Design review of the part built by this model. Coordinates are the model's own, in mm. A direction names the side the tool comes from. Give positions to 0.01 mm unless a question says otherwise; leave off trailing zeros. Order: outer loops, then holes, each group sorted by start corner. A loop starts at its lowest first (then second) coordinate and runs counter-clockwise, first axis right, second up. Notation, with made-up numbers: (16.25, 37.5) -> (42.25, 37.5) arc R7 cw to (42.25, 47.5) -> close; hole circle Ø11 at (42, 53). An arc over 180 degrees is marked (long way). One line per item, written item: value.
from build123d import *

# Parameters (mm, degrees)
SKETCH_1_W               = 45
SKETCH_1_H               = 12
EXTRUDE_1_DEPTH          = 4
SKETCH_2_W               = 12
SKETCH_2_H               = 12
EXTRUDE_2_DEPTH          = 15
SKETCH_3_W               = 2
SKETCH_3_H               = 10
EXTRUDE_3_DEPTH          = 2
SKETCH_4_W               = 21
SKETCH_4_H               = 21
EXTRUDE_4_DEPTH          = 19
SKETCH_5_W               = 13
SKETCH_5_H               = 13
CUT_EXTRUDE_1_DEPTH      = 50.782024868
SKETCH_6_W               = 13
SKETCH_6_H               = 4
CUT_EXTRUDE_2_DEPTH      = 12
CUT_EXTRUDE_3_REACH      = 54.671
SKETCH_7_W               = 5
SKETCH_7_H               = 2
CUT_EXTRUDE_4_REACH      = 54.671
SKETCH_8_R               = 1.5
CHAMFER_1_SIZE           = 2
CUT_EXTRUDE_5_DEPTH      = 50.053542176
CUT_EXTRUDE_5_DEPTH_BACK = 50.053542176
SKETCH_9_R               = 3.5
CUT_EXTRUDE_6_DEPTH      = 51.5791459
CUT_EXTRUDE_6_DEPTH_BACK = 2
SKETCH_10_R              = 2
CUT_EXTRUDE_7_DEPTH      = 50.782024868
CUT_EXTRUDE_7_DEPTH_BACK = 50.782024868
SKETCH_11_R              = 2
CUT_EXTRUDE_8_DEPTH      = 51.5791459
CUT_EXTRUDE_8_DEPTH_BACK = 10
SKETCH_12_R              = 3.5
SKETCH_13_W              = 21
SKETCH_13_H              = 7
CUT_EXTRUDE_9_DEPTH      = 17
SKETCH_14_R              = 3.5
EXTRUDE_5_DEPTH          = 4


with BuildPart() as part:
    # 草图1 → 凸台-拉伸1 (new body)
    with BuildSketch(Plane(origin=(0, 0, 0), x_dir=(1, 0, 0), z_dir=(0, 1, 0))):
        Rectangle(SKETCH_1_W, SKETCH_1_H)
    extrude(amount=EXTRUDE_1_DEPTH)

    # 草图2 → 凸台-拉伸2 (add)
    with BuildSketch(Plane(origin=(0, 4, 0), x_dir=(1, 0, 0), z_dir=(0, 1, 0))):
        with Locations((16.5, 0)):
            Rectangle(SKETCH_2_W, SKETCH_2_H)
    extrude(amount=EXTRUDE_2_DEPTH)

    # 草图3 → 凸台-拉伸3 (add)
    with BuildSketch(Plane(origin=(0, 19, 0), x_dir=(1, 0, 0), z_dir=(0, 1, 0))):
        with Locations((11.5, 0)):
            Rectangle(SKETCH_3_W, SKETCH_3_H)
        with Locations((21.5, 0)):
            Rectangle(SKETCH_3_W, SKETCH_3_H)
    extrude(amount=EXTRUDE_3_DEPTH)

    # 草图4 → 凸台-拉伸4 (add)
    with BuildSketch(Plane.XZ):
        with Locations((33, -4.5)):
            Rectangle(SKETCH_4_W, SKETCH_4_H)
    extrude(amount=-EXTRUDE_4_DEPTH)

    # 草图5 → 切除-拉伸1 (cut, through all)
    with BuildSketch(Plane(origin=(0, 19, 0), x_dir=(1, 0, 0), z_dir=(0, 1, 0))):
        with Locations((33, 4.5)):
            Rectangle(SKETCH_5_W, SKETCH_5_H)
    extrude(amount=-CUT_EXTRUDE_1_DEPTH, mode=Mode.SUBTRACT)

    # 草图6 → 切除-拉伸2 (cut)
    with BuildSketch(Plane(origin=(0, 19, 0), x_dir=(1, 0, 0), z_dir=(0, 1, 0))):
        with Locations((33, -4)):
            Rectangle(SKETCH_6_W, SKETCH_6_H)
    extrude(amount=-CUT_EXTRUDE_2_DEPTH, mode=Mode.SUBTRACT)

    # 草图7 → 切除-拉伸3 (cut, up to next)
    with BuildSketch(Plane.XY.offset(6), mode=Mode.PRIVATE) as cut_extrude_3_sk1:
        with Locations((33, 7)):
            Rectangle(SKETCH_7_W, SKETCH_7_H)
    cut_extrude_3_tool1 = extrude(cut_extrude_3_sk1.sketch, amount=-CUT_EXTRUDE_3_REACH, mode=Mode.PRIVATE) & part.part
    add(cut_extrude_3_tool1.solids().sort_by_distance((33, 7, 6))[0], mode=Mode.SUBTRACT)

    # 草图8 → 切除-拉伸4 (cut, up to next)
    with BuildSketch(Plane.XY.offset(6), mode=Mode.PRIVATE) as cut_extrude_4_sk1:
        with Locations((33, 4)):
            Circle(SKETCH_8_R)
    cut_extrude_4_tool1 = extrude(cut_extrude_4_sk1.sketch, amount=-CUT_EXTRUDE_4_REACH, mode=Mode.PRIVATE) & part.part
    add(cut_extrude_4_tool1.solids().sort_by_distance((33, 4, 6))[0], mode=Mode.SUBTRACT)

    # 倒角1
    chamfer_1_edges = [part.edges().sort_by_distance(p)[0] for p in [
        (-22.5, 2, -6),
        (-22.5, 2, 6),
    ]]
    chamfer(chamfer_1_edges, length=CHAMFER_1_SIZE)

    # 草图9 → 切除-拉伸5 (cut, two sides: drawn at the far end of the back side and taken through both)
    with BuildSketch(Plane(origin=(0, 4, 0), x_dir=(1, 0, 0), z_dir=(0, 1, 0)).offset(-CUT_EXTRUDE_5_DEPTH_BACK)):
        with Locations(Location((-15.5, 0, 0), (0, 0, 270))):
            Circle(SKETCH_9_R)
    extrude(amount=CUT_EXTRUDE_5_DEPTH + CUT_EXTRUDE_5_DEPTH_BACK, mode=Mode.SUBTRACT)

    # 草图10 → 切除-拉伸6 (cut, two sides: drawn at the far end of the back side and taken through both)
    with BuildSketch(Plane.XZ.offset(-CUT_EXTRUDE_6_DEPTH_BACK)):
        with BuildLine():
            Line((8.625, 1.996089928), (-15.28125, 3.493157374))
            ThreePointArc((-15.28125, 3.493157374), (-12.948958546, 2.396286189), (-12, 0))
            ThreePointArc((-12, 0), (-12.948958546, -2.396286189), (-15.28125, -3.493157374))
            Line((-15.28125, -3.493157374), (8.625, -1.996089928))
            ThreePointArc((8.625, -1.996089928), (6.5, 0), (8.625, 1.996089928))
        make_face()
        with Locations((8.5, 0)):
            Circle(SKETCH_10_R)
    extrude(amount=CUT_EXTRUDE_6_DEPTH + CUT_EXTRUDE_6_DEPTH_BACK, mode=Mode.SUBTRACT)

    # 草图11 → 切除-拉伸7 (cut, two sides: drawn at the far end of the back side and taken through both)
    with BuildSketch(Plane(origin=(0, 19, 0), x_dir=(1, 0, 0), z_dir=(0, 1, 0)).offset(-CUT_EXTRUDE_7_DEPTH_BACK)):
        with Locations(Location((16.5, 0, 0), (0, 0, 270))):
            Circle(SKETCH_11_R)
    extrude(amount=CUT_EXTRUDE_7_DEPTH + CUT_EXTRUDE_7_DEPTH_BACK, mode=Mode.SUBTRACT)

    # 草图12 → 切除-拉伸8 (cut, two sides: drawn at the far end of the back side and taken through both)
    with BuildSketch(Plane.XZ.offset(-CUT_EXTRUDE_8_DEPTH_BACK)):
        with Locations(Location((16.5, 0, 0), (0, 0, 90))):
            Circle(SKETCH_12_R)
    extrude(amount=CUT_EXTRUDE_8_DEPTH + CUT_EXTRUDE_8_DEPTH_BACK, mode=Mode.SUBTRACT)

    # 草图13 → 切除-拉伸9 (cut)
    with BuildSketch(Plane(origin=(0, 0, -15), x_dir=(-1, 0, 0), z_dir=(0, 0, -1))):
        with Locations((-33, 3.5)):
            Rectangle(SKETCH_13_W, SKETCH_13_H)
    extrude(amount=-CUT_EXTRUDE_9_DEPTH, mode=Mode.SUBTRACT)

    # 草图14 → 凸台-拉伸5 (add)
    with BuildSketch(Plane(origin=(0, 0, -15), x_dir=(-1, 0, 0), z_dir=(0, 0, -1))):
        with Locations((-33, 13)):
            Circle(SKETCH_14_R)
    extrude(amount=EXTRUDE_5_DEPTH)


solid = part.part
Item 1: To check wall thickness, follow line 1 along X through (y, z) = (3.1, 0); line 2 along X through (y, z) = (14, 0); line 3 along Z through (x, y) = (16.5, 12.25). State the ranges of each line that lie inside material, in increasing order. Write a range as from..to.
Returned:
line 1: -22.5..-19, -12..13, 20..22.5
line 2: 10.5..14.5, 18.5..26.5, 39.5..43.5
line 3: -6..-2, 2..6
Item 2: Add section D-D on y = 14.5. Give the boundary of the cut face in (x, z), plus the area to 3 significant figures.
Returned:
outline: (10.5, -6) -> (22.5, -6) -> (22.5, -15) -> (29.84, -15) -> (29.84, -19) -> (36.16, -19) -> (36.16, -15) -> (43.5, -15) -> (43.5, 6) -> (39.5, 6) -> (39.5, -11) -> (26.5, -11) -> (26.5, 6) -> (10.5, 6) -> close; hole circle Ø4 at (16.5, 0)
area: 377 mm²
Item 3: Add section B-B on z = -8.75. Give the boundary of the cut face in (x, y), plus the area to 3 significant figures.
Returned:
outline: (22.5, 7) -> (26.5, 7) -> (26.5, 19) -> (22.5, 19) -> close; (39.5, 7) -> (43.5, 7) -> (43.5, 19) -> (39.5, 19) -> close
area: 96.0 mm²
Item 4: Machinability: for faces 1 (the flat face through (22.5, 3, -2)), 2 (the flat face through (12.5, 20, 0)), 3 (the flat face through (11, 20, 5)), 4 (the flat face through (-6, 4, 0)), which of the approach directions +Z, -Z, +X, -X, +Y, -Y give a long, thin tool a straight path to every point of the face, cutting with its end or side? Answer none if there is none.
Returned:
face 1: -Z, +X, -Y
face 2: +Z, -Z, +Y
face 3: +Z, +X, -X, +Y
face 4: +Z, -Z, -X, +Y
Item 5: Draft analysis for pull direction Z (two halves, no side actions). For faces 5 (the flat face through (30.5, 10.2, -15)), 6 (the flat face through (18, 10, 2)), 7 (the cylindrical face through (-18.917, 2.416, -0.759)), 8 (the flat face through (22.5, 13, -11)), state which applies: pulls with the +Z half, pulls with the -Z half, needs draft (parallel to the pull), parting line crosses it, or undercut.
Returned:
face 5: pulls with the -Z half
face 6: undercut
face 7: undercut
face 8: needs draft
Item 6: Add section A-A on x = 33. Give the boundary of the cut face in (y, z).
Returned:
outline: (0, 2) -> (2.5, 2) -> (2.5, 6) -> (0, 6) -> close; (5.5, 2) -> (6, 2) -> (6, 6) -> (5.5, 6) -> close; (7, -15) -> (9.5, -15) -> (9.5, -19) -> (16.5, -19) -> (16.5, -15) -> (19, -15) -> (19, -11) -> (7, -11) -> close
Item 7: Add section C-C on z = 0. Count the separate pieces of the cut face and the enclosed holes in it, plus the area to 3 significant figures.
Returned:
separate pieces: 4
enclosed holes: 0
area: 285 mm²
Item 8: Clearance check with flat-ended pins moving along their axes: P1, Ø5.5, axis at x = 16.5, z = 0, coming from the -Y side; P2, Ø4, axis at x = -7, y = 5.5, coming from the -Z side; P3, Ø8, axis at y = 14, z = 1.5, coming from the -X side. State where each tip first meets the part, or that it passes through.
Returned:
P1: y = 10
P2: z = -6
P3: x = 10.5
